```python
from build123d import *

# Parameters (mm, degrees)
F0_W     = 45.72
F0_H     = 83.312
F1_DEPTH = 2.54
F2_W     = 45.72
F2_H     = 83.312
F2_W_2   = 40.64
F2_H_2   = 78.232
F3_DEPTH = 20.32
F4_R     = 1.27
F4_R_2   = 2.54
F4_W     = 31.75
F4_H     = 3.175
F5_DEPTH = 25.4


with BuildPart() as f1:
    # F0 (on Top) → F1 (new body)
    with BuildSketch(Plane.XY):
        Rectangle(F0_W, F0_H)
    extrude(amount=F1_DEPTH)

    # F2 (on face) → F3 (join)
    with BuildSketch(Plane.XY.offset(2.54)):
        Rectangle(F2_W, F2_H)
        Rectangle(F2_W_2, F2_H_2, mode=Mode.SUBTRACT)
    extrude(amount=F3_DEPTH)

    # F4 (on face) → F5 (cut)
    with BuildSketch(Plane.XY.offset(2.54)):
        with Locations((0, 28.702)):
            Circle(F4_R)
        with Locations((0, -28.702)):
            Circle(F4_R)
        with Locations((17.78, 28.702)):
            Circle(F4_R_2)
        with Locations((-17.78, -28.702)):
            Circle(F4_R_2)
        with Locations((0, 37.5285)):
            Rectangle(F4_W, F4_H)
        with Locations((0, -37.5285)):
            Rectangle(F4_W, F4_H)
    extrude(amount=-F5_DEPTH, mode=Mode.SUBTRACT)


solid = f1.part
```
Part model, mm, in its own coordinate system. A direction names the side the tool comes from. Give positions to 0.01 mm unless a question says otherwise; leave off trailing zeros. Order: outer loops, then holes, each group sorted by start corner. A loop starts at its lowest first (then second) coordinate and runs counter-clockwise, first axis right, second up. Notation, with made-up numbers: M 49,34.5 L 53,34.5 A13 cw 53,51.5 Z; hole C 31,27.5 d10. An arc over 180 degrees is marked long. Use a Markdown table: item, result. Add a question column.
(1) Probe line 1 along Y through (x, z) = (0, 1.6); line 2 along Y through (x, z) = (17.78, 0.9); line 3 along X through (y, z) = (-2, 13.5). List the from-to ranges inside material, lowest first. Write a range as [from, to].
(2) 3-axis set-ups, long thin cutter, end or side, ignore diameter. For faces 5 (the face through (0, -41.656, 11)), 6 (the face through (15.875, -38, 1)), 7 (the face through (0, -39.116, 11)): which of +Z, -Z, +X, -X, +Y, -Y reach the whole face in a straight line?
(3) Saw through at A-A, the plane x = 3.5. Give the cut face in (y, z), and give its area (3 significant figures).
(4) Saw through at D-D, the plane y = -12. Give the cut face in (x, z), and give its area (3 significant figures).
(5) Mould opens along X. For faces 1 (the face through (0, 1, 0)), 2 (the face through (-0.275, 27.462, 1.288)), 3 (the face through (-22.86, -1, 11)), 4 (the face through (0, 1, 2.54)) say: +X half, -X half, draft (parallel to the pull), parting line (faces both ways), or undercut.
(6) Drop flat-ended pins along their axis: P1, Ø3.5, axis at x = 0, y = 28.702, coming from the +Z side; P2, Ø4, axis at x = -17.78, y = -28.702, coming from the +Z side. Give the stop position or say it passes through.
(7) Saw through at B-B, the plane x = -17.78. Give the cut face in (y, z).
(8) Saw through at C-C, the plane z = 4.25. Give the cut face in (x, y), and give its area (3 significant figures).
Answer key:
| question | item | result |
|---|---|---|
| 1 | line 1 | [-41.66, -39.12], [-35.94, -29.97], [-27.43, 27.43], [29.97, 35.94], [39.12, 41.66] |
| 1 | line 2 | [-41.66, 26.16], [31.24, 41.66] |
| 1 | line 3 | [-22.86, -20.32], [20.32, 22.86] |
| 2 | face 5 | +Z, -Z, +X, -X, -Y |
| 2 | face 6 | +Z, -Z |
| 2 | face 7 | +Z |
| 3 | outline | M -41.66,0 L -39.12,0 L -39.12,22.86 L -41.66,22.86 Z; M -35.94,0 L 35.94,0 L 35.94,2.54 L -35.94,2.54 Z; M 39.12,0 L 41.66,0 L 41.66,22.86 L 39.12,22.86 Z |
| 3 | area | 299 mm^2 |
| 4 | outline | M -22.86,0 L 22.86,0 L 22.86,22.86 L 20.32,22.86 L 20.32,2.54 L -20.32,2.54 L -20.32,22.86 L -22.86,22.86 Z |
| 4 | area | 219 mm^2 |
| 5 | face 1 | draft |
| 5 | face 2 | undercut |
| 5 | face 3 | -X half |
| 5 | face 4 | undercut |
| 6 | P1 | z = 2.54 |
| 6 | P2 | through |
| 7 | outline | M -41.66,0 L -31.24,0 L -31.24,2.54 L -39.12,2.54 L -39.12,22.86 L -41.66,22.86 Z; M -26.16,0 L 41.66,0 L 41.66,22.86 L 39.12,22.86 L 39.12,2.54 L -26.16,2.54 Z |
| 8 | outline | M -22.86,-41.66 L 22.86,-41.66 L 22.86,41.66 L -22.86,41.66 Z; hole M -20.32,-39.12 L 20.32,-39.12 L 20.32,39.12 L -20.32,39.12 Z |
| 8 | area | 630 mm^2 |
